from build123d import *

# Parameters (mm, degrees)
RESSALTO_EXTRUS_O1_DEPTH                   = 8
BROCA_DE_ROSQUEAR_PARA_TARRAXA_DE_M6X1_0_D = 5
RESSALTO_EXTRUS_O2_DEPTH                   = 30
ESBO_O6_W                                  = 10
ESBO_O6_H                                  = 40
ESBO_O6_H_2                                = 25
CORTE_EXTRUS_O2_DEPTH                      = 20
ESBO_O14_R                                 = 3
CORTE_EXTRUS_O6_DEPTH                      = 39
ESBO_O15_R                                 = 4.25
CORTE_EXTRUS_O7_DEPTH                      = 40
RESSALTO_EXTRUS_O3_DEPTH                   = 10
ESBO_O17_W                                 = 9.5
ESBO_O17_H                                 = 40
RESSALTO_EXTRUS_O4_DEPTH                   = 30
ESBO_O18_R                                 = 2.5
CORTE_EXTRUS_O8_DEPTH                      = 10
ESBO_O19_W                                 = 60
ESBO_O19_H                                 = 9.5
RESSALTO_EXTRUS_O5_DEPTH                   = 30
FILETE1_R                                  = 5
ESBO_O20_R                                 = 2.5
CORTE_EXTRUS_O9_DEPTH                      = 10


with BuildPart() as part:
    # Esboço1 → Ressalto-extrusão1 (new body)
    with BuildSketch(Plane.XY):
        with BuildLine():
            Line((440, 72.212171493), (380, 72.212171493))
            Line((380, 72.212171493), (380, 132.212171493))
            ThreePointArc((380, 132.212171493), (382.928932188, 139.283239304), (390, 142.212171493))
            Line((390, 142.212171493), (470, 142.212171493))
            Line((470, 142.212171493), (470, 102.212171493))
            Line((470, 102.212171493), (440, 102.212171493))
            Line((440, 102.212171493), (440, 72.212171493))
        make_face()
    extrude(amount=RESSALTO_EXTRUS_O1_DEPTH)

    # Broca de rosquear para tarraxa de M6x1.01 (through all)
    with Locations(Plane.XY.offset(8)):
        with Locations((393, 87.212171493), (427, 87.212171493), (455, 112.212171493), (455, 132.212171493)):
            Hole(BROCA_DE_ROSQUEAR_PARA_TARRAXA_DE_M6X1_0_D / 2)

    # Esboço4 → Ressalto-extrusão2 (add)
    with BuildSketch(Plane(origin=(0, 0, 0), x_dir=(-1, 0, 0), z_dir=(0, 0, -1))):
        with BuildLine():
            Line((-390, 142.212171493), (-440, 142.212171493))
            Line((-440, 142.212171493), (-440, 102.212171493))
            Line((-440, 102.212171493), (-380, 102.212171493))
            Line((-380, 102.212171493), (-380, 132.212171493))
            ThreePointArc((-380, 132.212171493), (-382.928932188, 139.283239304), (-390, 142.212171493))
        make_face()
    extrude(amount=RESSALTO_EXTRUS_O2_DEPTH)

    # Esboço6 → Corte-extrusão2 (cut)
    with BuildSketch(Plane.ZY.offset(-380)):
        with Locations((-22.874860756, 122.212171493)):
            Rectangle(ESBO_O6_W, ESBO_O6_H)
        with Locations((-8.874860756, 129.712171493)):
            Rectangle(ESBO_O6_W, ESBO_O6_H_2)
    extrude(amount=-CORTE_EXTRUS_O2_DEPTH, mode=Mode.SUBTRACT)

    # Esboço14 → Corte-extrusão6 (cut, through all)
    with BuildSketch(Plane(origin=(0, 0, -30), x_dir=(-1, 0, 0), z_dir=(0, 0, -1))):
        with Locations((-390, 129.712171493)):
            Circle(ESBO_O14_R)
        with Locations((-390, 114.712171493)):
            Circle(ESBO_O14_R)
    extrude(amount=-CORTE_EXTRUS_O6_DEPTH, mode=Mode.SUBTRACT)

    # Esboço15 → Corte-extrusão7 (cut)
    with BuildSketch(Plane(origin=(0, 142.212171493, 0), x_dir=(1, 0, 0), z_dir=(0, 1, 0))):
        with Locations((420, 18.90241208)):
            Circle(ESBO_O15_R)
        with Locations((420, 1.90241208)):
            Circle(ESBO_O15_R)
    extrude(amount=-CORTE_EXTRUS_O7_DEPTH, mode=Mode.SUBTRACT)


with BuildPart() as body_2:
    # Espelhar1: mirrored copy
    add(part.part.mirror(Plane(origin=(380, 72.212171493, 8), x_dir=(0, 0, 1), z_dir=(-1, 0, 0))))

    # Esboço16 → Ressalto-extrusão3 (add)
    with BuildSketch(Plane(origin=(0, 0, -30), x_dir=(-1, 0, 0), z_dir=(0, 0, -1))):
        with BuildLine():
            Line((-320, 142.212171493), (-328, 142.212171493))
            Line((-328, 142.212171493), (-328, 110.212171493))
            Line((-328, 110.212171493), (-365.320990692, 110.212171493))
            ThreePointArc((-365.320990692, 110.212171493), (-369.387979043, 108.52756976), (-373.454967393, 110.212171493))
            Line((-373.454967393, 110.212171493), (-380, 110.212171493))
            Line((-380, 110.212171493), (-380, 102.212171493))
            Line((-380, 102.212171493), (-328, 102.212171493))
            Line((-328, 102.212171493), (-320, 102.212171493))
            Line((-320, 102.212171493), (-320, 142.212171493))
        make_face()
    extrude(amount=RESSALTO_EXTRUS_O3_DEPTH)

    # Esboço17 → Ressalto-extrusão4 (add, through all)
    with BuildSketch(Plane.ZY.offset(-320)):
        with Locations((-35.25, 122.212171493)):
            Rectangle(ESBO_O17_W, ESBO_O17_H)
    extrude(amount=RESSALTO_EXTRUS_O4_DEPTH)

    # Esboço18 → Corte-extrusão8 (cut)
    with BuildSketch(Plane.XY.offset(-30.5)):
        with Locations((305, 112.212171493)):
            Circle(ESBO_O18_R)
        with Locations((305, 132.212171493)):
            Circle(ESBO_O18_R)
    extrude(amount=-CORTE_EXTRUS_O8_DEPTH, mode=Mode.SUBTRACT)

    # Esboço19 → Ressalto-extrusão5 (add, through all)
    with BuildSketch(Plane.XZ.offset(-102.212171493)):
        with Locations((350, -35.25)):
            Rectangle(ESBO_O19_W, ESBO_O19_H)
    extrude(amount=RESSALTO_EXTRUS_O5_DEPTH)

    # Filete1
    filete1_edges = [body_2.edges().sort_by_distance(p)[0] for p in [
        (328, 110.212171493, -35),
    ]]
    fillet(filete1_edges, radius=FILETE1_R)

    # Esboço20 → Corte-extrusão9 (cut)
    with BuildSketch(Plane.XY.offset(-30.5)):
        with Locations((367, 87.212171493)):
            Circle(ESBO_O20_R)
        with Locations((333, 87.212171493)):
            Circle(ESBO_O20_R)
    extrude(amount=-CORTE_EXTRUS_O9_DEPTH, mode=Mode.SUBTRACT)


solid = body_2.part
Check sheet for the modelled part. Datum: model origin and axes. Units: mm. A direction names the side the tool comes from. Round coordinates to 2 decimals unless told otherwise and drop trailing zeros. Loops run counter-clockwise (first coordinate to the right, second up) from the corner with the lowest first, then second, coordinate; pieces in that order, holes last. Notation, with made-up numbers: M 35,84 L 75,84 A23 ccw 75,107 Z; hole C -26.75,33.5 d2. An arc over 180 degrees is marked long. One line per question, with ' | ' between items. Start each with the question number.
Item 1: Scan lines: probe 1 along Z at (x, y) = (340, 117); probe 2 along Z at (x, y) = (311.5, 116); probe 3 along X at (y, z) = (112.5, -17). Record each from-to range of solid material in increasing order.
Item 2: Set-up check for faces 1 (the face through (344.246, 122.492, -2.089)), 2 (the face through (369.325, 108.528, -34.93)), 3 (the face through (377, 110.212, -35)): record each of +Z, -Z, +X, -X, +Y, -Y from which the full face is reachable in a straight line by a thin tool's end or side.
Item 3: Section check A-A (y = 97). Record the boundary of the cut face in (x, z), and give its area (3 significant figures).
Item 4: Section check B-B (x = 340). Record the boundary of the cut face in (y, z), and give its area (4 significant figures).
Item 5: Release check for a two-part mould opening along Z. For faces 4 (the face through (307.385, 132.963, -35.184)), 5 (the face through (370, 122, -17.875)) record: released by +Z, released by -Z, zero draft, split by the parting line, or undercut.
Item 6: Gauge pin test, flat ends, axial feed: pin 1 Ø22 at (x, y) = (368.5, 127.5) entering from -Z; pin 2 Ø6.5 at (x, y) = (305, 112.21) entering from +Z; pin 3 Ø3 at (x, y) = (367, 87.21) entering from +Z (3 decimals); pin 4 Ø0.7 at (x, z) = (342, 1) entering from +Y. Record the tip position at first contact, or that the pin passes through.
Item 7: Section check C-C (x = 305). Record the boundary of the cut face in (y, z).
Item 8: Section check D-D (z = -21). Record the boundary of the cut face in (x, y), and give its area (3 significant figures).
Worked out:
1) probe 1: -30 to -23.15, -14.65 to -6.15, 2.35 to 8 | probe 2: -40 to -30.5, 0 to 8 | probe 3: 320 to 336.2, 343.8 to 367.97, 372.03 to 380
2) face 1: +Y | face 2: -Z, +Y | face 3: -Z, +X, +Y
3) outline: M 320,-40 L 380,-40 L 380,-30.5 L 320,-30.5 Z; M 320,0 L 380,0 L 380,8 L 320,8 Z | area: 1,050 mm^2
4) outline: M 72.21,-40 L 110.21,-40 L 110.21,-30 L 142.21,-30 L 142.21,-23.15 L 102.21,-23.15 L 102.21,-30.5 L 72.21,-30.5 Z; M 72.21,0 L 102.21,0 L 102.21,2.35 L 142.21,2.35 L 142.21,8 L 72.21,8 Z; M 102.21,-14.65 L 142.21,-14.65 L 142.21,-6.15 L 102.21,-6.15 Z | area: 1,445 mm^2
5) face 4: zero draft | face 5: undercut
6) pin 1: z = -30 | pin 2: z = 8 | pin 3: through | pin 4: y = 102.21
7) outline: M 102.21,-40 L 109.71,-40 L 109.71,-30.5 L 102.21,-30.5 Z; M 102.21,0 L 109.71,0 L 109.71,8 L 102.21,8 Z; M 114.71,-40 L 129.71,-40 L 129.71,-30.5 L 114.71,-30.5 Z; M 114.71,0 L 129.71,0 L 129.71,8 L 114.71,8 Z; M 134.71,-40 L 142.21,-40 L 142.21,-30.5 L 134.71,-30.5 Z; M 134.71,0 L 142.21,0 L 142.21,8 L 134.71,8 Z
8) outline: M 320,102.21 L 336.3,102.21 L 336.3,142.21 L 320,142.21 Z; M 343.7,102.21 L 360,102.21 L 360,142.21 L 343.7,142.21 Z | area: 1,300 mm^2
